Part model, mm, in its own coordinate system. Give positions to 0.01 mm unless a question says otherwise; leave off trailing zeros. Order: outer loops, then holes, each group sorted by start corner. A loop starts at its lowest first (then second) coordinate and runs counter-clockwise, first axis right, second up.
1. Slice it at A-A on x = 5. List the corners of the cut face in (y, z), and give its area (3 significant figures).
2. Slice it at D-D on x = -7.5. List the corners of the cut face in (y, z).
3. Slice it at C-C on z = 41.5. List the corners of the cut face in (x, y), and give its area (3 significant figures).
4. Slice it at B-B on y = -1.65. List the corners of the cut face in (x, z).
5. Probe line 1 (Z direction, x = -0.5, y = -3.7); line 2 (X direction, y = -1.1, z = -2); line 3 (X direction, y = -2.45, z = 40.5). List the from-to ranges inside material, lowest first.
6. Drop flat-ended pins along their axis: pin 1 Ø2.5 at (x, y) = (10.5, -2) entering from +Z; pin 2 Ø7 at (x, z) = (5, 53.32) entering from +Y; pin 3 Ø1.5 at (x, y) = (-22, -1.5) entering from -Z; pin 4 Ø2 at (y, z) = (-1.5, -12) entering from -X. Give the stop position or say it passes through.
from build123d import *

# Parameters (mm, degrees)
F1_DEPTH = 5


with BuildPart() as f1:
    # F0 (on Front) → F1 (new body)
    with BuildSketch(Plane.XZ):
        Polygon((10, 10), (10, 50), (12.5, 52.5), (7.707753, 52.5), (7.063372, 52.5), (2.936628, 52.5), (2.292247, 52.5), (-2.5, 52.5), (0, 50), (0, 10), (-40, 10), (-42.5, 12.5), (-42.5, -2.5), (-40, 0), (0, 0), (0, -40), (10, -40), (10, 0), (50, 0), (52.5, -2.5), (52.5, 12.5), (50, 10), align=None)
        with BuildLine():
            Line((7.063372, 52.5), (7.707753, 52.5))
            ThreePointArc((7.707753, 52.5), (5, 56.455801), (2.292247, 52.5))
            Line((2.292247, 52.5), (2.936628, 52.5))
            ThreePointArc((2.936628, 52.5), (5, 55.540565), (7.063372, 52.5))
        make_face()
        Polygon((12.5, -42.5), (10, -40), (0, -40), (-2.5, -42.5), align=None)
    extrude(amount=F1_DEPTH)


solid = f1.part
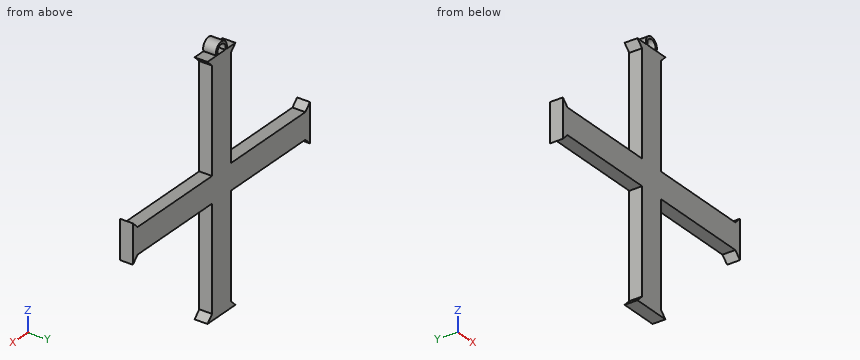
Data:
1. outline: (-5, -42.5) - (0, -42.5) - (0, 52.5) - (-5, 52.5) - close; (-5, 55.54) - (0, 55.54) - (0, 56.46) - (-5, 56.46) - close
1. area: 480 mm2
2. outline: (-5, 0) - (0, 0) - (0, 10) - (-5, 10) - close
3. outline: (0, -5) - (10, -5) - (10, 0) - (0, 0) - close
3. area: 50.0 mm2
4. outline: (-42.5, -2.5) - (-40, 0) - (0, 0) - (0, -40) - (-2.5, -42.5) - (12.5, -42.5) - (10, -40) - (10, 0) - (50, 0) - (52.5, -2.5) - (52.5, 12.5) - (50, 10) - (10, 10) - (10, 50) - (12.5, 52.5) - (7.71, 52.5) arc R2.9 ccw (long way) to (2.29, 52.5) - (-2.5, 52.5) - (0, 50) - (0, 10) - (-40, 10) - (-42.5, 12.5) - close; hole (2.94, 52.5) - (7.06, 52.5) arc R2.22 ccw (long way) to start
5. line 1: z = -42.5 to -40.5, 0 to 10, 50.5 to 52.5
5. line 2: x = -42.5 to -42, 0 to 10, 52 to 52.5
5. line 3: x = 0 to 10
6. pin 1: stops at z = 52.5
6. pin 2: stops at y = 0
6. pin 3: stops at z = 0
6. pin 4: stops at x = 0
